```python
from build123d import *

# Parameters (mm, degrees)
F2_R     = 2.54
F3_DEPTH = 25.4


with BuildPart() as f1:
    # F0 (on Right) → F1 (revolve)
    with BuildSketch(Plane.YZ):
        Polygon((31.75, 12.7), (31.75, 0), (38.1, 0), (38.1, 19.05), (27.94, 19.05), (27.94, 12.7), align=None)
    revolve(axis=Axis((0, 0, 13.59911), (0, 0, 1)))

    # F2 (on face) → F3 (cut)
    with BuildSketch(Plane.XY.offset(19.05)):
        with Locations((-34.925, 0)):
            Circle(F2_R)
        with Locations((0, 34.925)):
            Circle(F2_R)
        with Locations((34.925, 0)):
            Circle(F2_R)
        with Locations((0, -34.925)):
            Circle(F2_R)
    extrude(amount=-F3_DEPTH, mode=Mode.SUBTRACT)


solid = f1.part
```
Can you work these out from the model? Positions are in its coordinate system, mm. A direction names the side the tool comes from. Give positions to 0.01 mm unless a question says otherwise; leave off trailing zeros. Order: outer loops, then holes, each group sorted by start corner. A loop starts at its lowest first (then second) coordinate and runs counter-clockwise, first axis right, second up. Notation, with made-up numbers: (17, 81.5) - (75, 81.5) arc R15 cw to (75, 97.5) - close; hole circle Ø1 at (19.5, 83.25). An arc over 180 degrees is marked (long way). Use a Markdown table: item, result. Add a question column.
Q1. On a 3-axis mill with a long thin cutter (end or side, diameter ignored), from which of +Z, -Z, +X, -X, +Y, -Y can I reach the whole of each face in a straight line? I mean faces 4 (the cylindrical face through (-27.7, -3.64, 15.83)), 5 (the cylindrical face through (30.995, -6.883, 6.261)). Say none if no direction works.
Q2. If we mould it in two halves opening along X, with no side actions, what happens to faces 1 (the flat face through (-23, 23, 0)), 2 (the flat face through (28.1, 0.1, 12.7)), 3 (the cylindrical face through (23.183, -30.235, 9.658))? For each: released by +X, released by -X, zero draft, split by the parting line, or undercut.
Q3. If we section it at C-C on y = 20: Write out the boundary of the cut face in (x, z), plus the area to 3 significant figures.
Q4. If we section it at A-A on y = 0: Write out the boundary of the cut face in (x, z) (3 decimals), plus the area to 3 significant figures.
Q5. Please list where these lines run through material, in increasing order: line 1 along Y through (x, z) = (0, 7.75) (3 decimals); line 2 along Y through (x, z) = (1, 15.75); line 3 along X through (y, z) = (-10, 6.75).
Q6. I'm going to push flat-ended pins straight in: pin 1 (5 mm diameter, centred on x = 10, y = 21.5, fed in from -Z); pin 2 (8 mm diameter, centred on y = -14, z = 14.5, fed in from -X); pin 3 (2 mm diameter, centred on y = 28.5, z = 10, fed in from +X); pin 4 (10 mm diameter, centred on y = 2.5, z = 16.5, fed in from +X). Where does each tip first touch, or does it pass through?
Q7. If we section it at D-D on z = 3: Write out the boundary of the cut face in (x, y) (3 decimals), plus the area to 3 significant figures.
Answers follow:
| question | item | result |
|---|---|---|
| 1 | face 4 | +Z, -Z |
| 1 | face 5 | -Z |
| 2 | face 1 | zero draft |
| 2 | face 2 | undercut |
| 2 | face 3 | split by the parting line |
| 3 | outline | (-32.43, 0) - (-24.66, 0) - (-24.66, 12.7) - (-19.51, 12.7) - (-19.51, 19.05) - (-32.43, 19.05) - close; (19.51, 12.7) - (24.66, 12.7) - (24.66, 0) - (32.43, 0) - (32.43, 19.05) - (19.51, 19.05) - close |
| 3 | area | 361 mm^2 |
| 4 | outline | (-38.1, 0) - (-37.465, 0) - (-37.465, 19.05) - (-38.1, 19.05) - close; (-32.385, 0) - (-31.75, 0) - (-31.75, 12.7) - (-27.94, 12.7) - (-27.94, 19.05) - (-32.385, 19.05) - close; (27.94, 12.7) - (31.75, 12.7) - (31.75, 0) - (32.385, 0) - (32.385, 19.05) - (27.94, 19.05) - close; (37.465, 0) - (38.1, 0) - (38.1, 19.05) - (37.465, 19.05) - close |
| 4 | area | 96.8 mm^2 |
| 5 | line 1 | y = -38.1 to -37.465, -32.385 to -31.75, 31.75 to 32.385, 37.465 to 38.1 |
| 5 | line 2 | y = -38.09 to -37.26, -32.59 to -27.92, 27.92 to 32.59, 37.26 to 38.09 |
| 5 | line 3 | x = -36.76 to -30.13, 30.13 to 36.76 |
| 6 | pin 1 | passes through |
| 6 | pin 2 | stops at x = -36.76 |
| 6 | pin 3 | stops at x = 26.37 |
| 6 | pin 4 | stops at x = 38.1 |
| 7 | outline | circle Ø76.2 at (0, 0); hole circle Ø5.08 at (-34.925, 0); hole circle Ø63.5 at (0, 0); hole circle Ø5.08 at (0, -34.925); hole circle Ø5.08 at (0, 34.925); hole circle Ø5.08 at (34.925, 0) |
| 7 | area | 1,310 mm^2 |
